Read the model definition and answer for the solid it produces. Units are mm, in the model's axes. Coordinates: 2 decimals unless noted, no trailing zeros. Loops run counter-clockwise (first coordinate to the right, second up) from the corner with the lowest first, then second, coordinate; pieces in that order, holes last.
from build123d import *

# Parameters (mm, degrees)
SKETCH2_R                  = 4.7625
BOSS_EXTRUDE1_DEPTH        = 76.2
F_10_32_TAPPED_HOLE1_D     = 4.0386
F_10_32_TAPPED_HOLE1_DEPTH = 15.24
F_10_32_TAPPED_HOLE1_TIP   = 1.213317848
F_6_32_TAPPED_HOLE1_D      = 2.7051
F_6_32_TAPPED_HOLE1_DEPTH  = 9.398
F_6_32_TAPPED_HOLE1_TIP    = 0.81269403


with BuildPart() as part:
    # Sketch2 → Boss-Extrude1 (new body)
    with BuildSketch(Plane.XY):
        with Locations(Location((0, 0, 0), (0, 0, 180))):
            Circle(SKETCH2_R)
    extrude(amount=BOSS_EXTRUDE1_DEPTH)

    # #10-32 Tapped Hole1
    with Locations(Plane(origin=(0, 0, 0), x_dir=(-1, 0, 0), z_dir=(0, 0, -1))):
        with Locations((-0.028702786, 0.067410108)):
            Hole(F_10_32_TAPPED_HOLE1_D / 2, depth=F_10_32_TAPPED_HOLE1_DEPTH)
            with Locations((0, 0, -(F_10_32_TAPPED_HOLE1_DEPTH + F_10_32_TAPPED_HOLE1_TIP / 2))):  # 118° drill point
                Cone(0, F_10_32_TAPPED_HOLE1_D / 2, F_10_32_TAPPED_HOLE1_TIP, mode=Mode.SUBTRACT)

    # #6-32 Tapped Hole1
    with Locations(Plane.XY.offset(76.2)):
        with Locations((0.02374074, -0.015572073)):
            Hole(F_6_32_TAPPED_HOLE1_D / 2, depth=F_6_32_TAPPED_HOLE1_DEPTH)
            with Locations((0, 0, -(F_6_32_TAPPED_HOLE1_DEPTH + F_6_32_TAPPED_HOLE1_TIP / 2))):  # 118° drill point
                Cone(0, F_6_32_TAPPED_HOLE1_D / 2, F_6_32_TAPPED_HOLE1_TIP, mode=Mode.SUBTRACT)


solid = part.part
Q1. Determine the mould class of faces 1 (the face through (1.03, 4.65, 37.57)), 2 (the face through (-2, 1, 0)), 3 (the face through (-0.409, -1.904, 7.727)), 4 (the face through (-1.266, 0.391, 71.435)) for opening direction X: +X half, -X half, draft (parallel to the pull), parting line (faces both ways), or undercut.
Findings below:
face 1: parting line
face 2: draft
face 3: undercut
face 4: undercut
Q2. A cutting plane is placed at B-B (y = 3.25). Give the vertices of the cut face in (x, z), then the cut area to 3 significant figures.
Findings below:
outline: (-3.48, 0) - (3.48, 0) - (3.48, 76.2) - (-3.48, 76.2) - close
area: 531 mm2
Q3. A cutting plane is placed at A-A (z = 32.5). Give the vertices of the cut face in (x, y) (1 decimal).
Findings below:
outline: circle Ø9.5 at (0, 0)
Q4. Straight lines are drawn through the part: probe 1 along Y at (x, z) = (-0.25, 26.5); probe 2 along X at (y, z) = (1, 12); probe 3 along Y at (x, z) = (1.25, 11.5). For each, find the intervals that lie inside material, in ascending order.
Findings below:
probe 1: y = -4.76 to 4.76
probe 2: x = -4.66 to -1.76, 1.82 to 4.66
probe 3: y = -4.6 to -1.54, 1.68 to 4.6
Q5. Flat-ended cylindrical pins translate along their axes: pin 1 Ø5 at (x, z) = (3, 30) entering from -Y; pin 2 Ø3 at (y, z) = (-2.5, 14) entering from -X; pin 3 Ø2.5 at (x, y) = (0.02, -0.02) entering from +Z. Find the tip coordinate at first contact, or state that the pin passes through.
Findings below:
pin 1: stops at y = -4.74
pin 2: stops at x = -4.66
pin 3: stops at z = 66.74
